```python
from build123d import *

# Parameters (mm, degrees)
SKETCH_1_R          = 35
SKETCH_1_R_2        = 9.5
EXTRUDE_1_DEPTH     = 18
SKETCH_2_R          = 40.856384021
SKETCH_2_R_2        = 11.482609949
CUT_EXTRUDE_1_DEPTH = 16
SKETCH_3_R          = 16.811419883
CUT_EXTRUDE_2_DEPTH = 10


with BuildPart() as part:
    # 草图1 → 凸台-拉伸1 (new body)
    with BuildSketch(Plane(origin=(0, 0, 0), x_dir=(1, 0, 0), z_dir=(0, 1, 0))):
        Circle(SKETCH_1_R)
        Circle(SKETCH_1_R_2, mode=Mode.SUBTRACT)
        with BuildLine():
            Line((19.832862473, 17.095228055), (8.333515071, 7.924804513))
            ThreePointArc((8.333515071, 7.924804513), (4.989663, 10.361141981), (1, 11.456439237))
            Line((1, 11.456439237), (1, 26.164656621))
            ThreePointArc((1, 26.164656621), (11.360707431, 23.59075206), (19.832862473, 17.095228055))
        make_face(mode=Mode.SUBTRACT)
        with BuildLine():
            Line((-1, 26.164656621), (-1, 11.456439237))
            ThreePointArc((-1, 11.456439237), (-4.989663, 10.361141981), (-8.333515071, 7.924804513))
            Line((-8.333515071, 7.924804513), (-19.832862473, 17.095228055))
            ThreePointArc((-19.832862473, 17.095228055), (-11.360707431, 23.59075206), (-1, 26.164656621))
        make_face(mode=Mode.SUBTRACT)
        with BuildLine():
            Line((21.079842076, 15.53156509), (9.580494675, 6.361141548))
            ThreePointArc((9.580494675, 6.361141548), (11.21167099, 2.55899074), (11.391723321, -1.574369647))
            Line((11.391723321, -1.574369647), (25.731174987, -4.847255916))
            ThreePointArc((25.731174987, -4.847255916), (25.527277881, 5.826434595), (21.079842076, 15.53156509))
        make_face(mode=Mode.SUBTRACT)
        with BuildLine():
            Line((25.286133119, -6.79711174), (10.946681453, -3.524225471))
            ThreePointArc((10.946681453, -3.524225471), (8.991062048, -7.170132721), (5.871731561, -9.888011351))
            Line((5.871731561, -9.888011351), (12.253387915, -23.139657316))
            ThreePointArc((12.253387915, -23.139657316), (20.471287425, -16.325306958), (25.286133119, -6.79711174))
        make_face(mode=Mode.SUBTRACT)
        with BuildLine():
            Line((10.45145018, -24.007424794), (4.069793825, -10.755778829))
            ThreePointArc((4.069793825, -10.755778829), (0, -11.5), (-4.069793825, -10.755778829))
            Line((-4.069793825, -10.755778829), (-10.45145018, -24.007424794))
            ThreePointArc((-10.45145018, -24.007424794), (0, -26.183759396), (10.45145018, -24.007424794))
        make_face(mode=Mode.SUBTRACT)
        with BuildLine():
            Line((-12.253387915, -23.139657316), (-5.871731561, -9.888011351))
            ThreePointArc((-5.871731561, -9.888011351), (-8.991062048, -7.170132721), (-10.946681453, -3.524225471))
            Line((-10.946681453, -3.524225471), (-25.286133119, -6.79711174))
            ThreePointArc((-25.286133119, -6.79711174), (-20.471287425, -16.325306958), (-12.253387915, -23.139657316))
        make_face(mode=Mode.SUBTRACT)
        with BuildLine():
            Line((-25.731174987, -4.847255916), (-11.391723321, -1.574369647))
            ThreePointArc((-11.391723321, -1.574369647), (-11.21167099, 2.55899074), (-9.580494675, 6.361141548))
            Line((-9.580494675, 6.361141548), (-21.079842076, 15.53156509))
            ThreePointArc((-21.079842076, 15.53156509), (-25.527277881, 5.826434595), (-25.731174987, -4.847255916))
        make_face(mode=Mode.SUBTRACT)
    extrude(amount=EXTRUDE_1_DEPTH)

    # 草图2 → 切除-拉伸1 (cut)
    with BuildSketch(Plane(origin=(0, 18, 0), x_dir=(1, 0, 0), z_dir=(0, 1, 0))):
        Circle(SKETCH_2_R)
        Circle(SKETCH_2_R_2, mode=Mode.SUBTRACT)
    extrude(amount=-CUT_EXTRUDE_1_DEPTH, mode=Mode.SUBTRACT)

    # 草图3 → 切除-拉伸2 (cut)
    with BuildSketch(Plane(origin=(0, 18, 0), x_dir=(1, 0, 0), z_dir=(0, 1, 0))):
        Circle(SKETCH_3_R)
    extrude(amount=-CUT_EXTRUDE_2_DEPTH, mode=Mode.SUBTRACT)


solid = part.part
```
Here's how the part is built. I have some questions about the finished solid (model axes, mm). Round coordinates to 2 decimals unless told otherwise and drop trailing zeros. Write each loop counter-clockwise with the first axis right and the second up, starting at its lowest first coordinate (ties: lowest second). Pieces come first, ordered by that corner, then holes. Notation, with made-up numbers: M 87,21.25 L 133,21.25 A21 cw 133,38.25 Z; hole C 22,-8 d1. An arc over 180 degrees is marked long. Answer as CSV lines item,"result". Start each with the question number.
1. Suppose I cut it at A-A on x = 0. Count the separate pieces of the cut face and the enclosed holes in it, then the cut area to 3 significant figures.
2. Thinking about a two-plate mould opening in Z: for faces 1 (the cylindrical face through (4.38, 3.94, 8.43)), 2 (the flat face through (-9.11, 0.99, 16.61)), 3 (the flat face through (-4, 8, -9)), which applies, released by +Z, released by -Z, zero draft, split by the parting line, or undercut?
3. Suppose I cut it at D-D on y = 5.25. Write out the boundary of the cut face in (x, z), then the cut area to 3 significant figures.
4. Suppose I cut it at C-C on x = -14.5. Write out the boundary of the cut face in (y, z).
5. I'm going to push flat-ended pins straight in: pin 1 Ø1 at (x, y) = (5, 4.5) entering from +Z; pin 2 Ø1 at (y, z) = (2, -1.5) entering from +X; pin 3 Ø1.6 at (y, z) = (1.5, -19) entering from +X; pin 4 Ø11.5 at (x, z) = (0, 0) entering from +Y. Where does each tip first touch, or does it pass through?
6. I need wall thicknesses on probe 1 along Z at (x, y) = (0, 5.5); probe 2 along X at (y, z) = (1.75, -23.5). Which ranges of each line are inside material? Lowest first, please.
Check result:
1,separate pieces,"3"
1,enclosed holes,"0"
1,area,"96.4 mm2"
2,face 1,"undercut"
2,face 2,"undercut"
2,face 3,"zero draft"
3,outline,"C 0,0 d22.97; hole C 0,0 d19"
3,area,"131 mm2"
4,outline,"M 0,-31.86 L 2,-31.86 L 2,-21.8 L 0,-21.8 Z; M 0,-12.84 L 2,-12.84 L 2,-10.28 L 0,-10.28 Z; M 0,2.28 L 2,2.28 L 2,4.34 L 0,4.34 Z; M 0,21.8 L 2,21.8 L 2,31.86 L 0,31.86 Z"
5,pin 1,"stops at z = 10.56"
5,pin 2,"stops at x = 34.99"
5,pin 3,"stops at x = 29.9"
5,pin 4,"passes through"
6,probe 1,"z = -11.48 to -9.5, 9.5 to 11.48"
6,probe 2,"x = -25.94 to -11.55, -1 to 1, 11.55 to 25.94"
